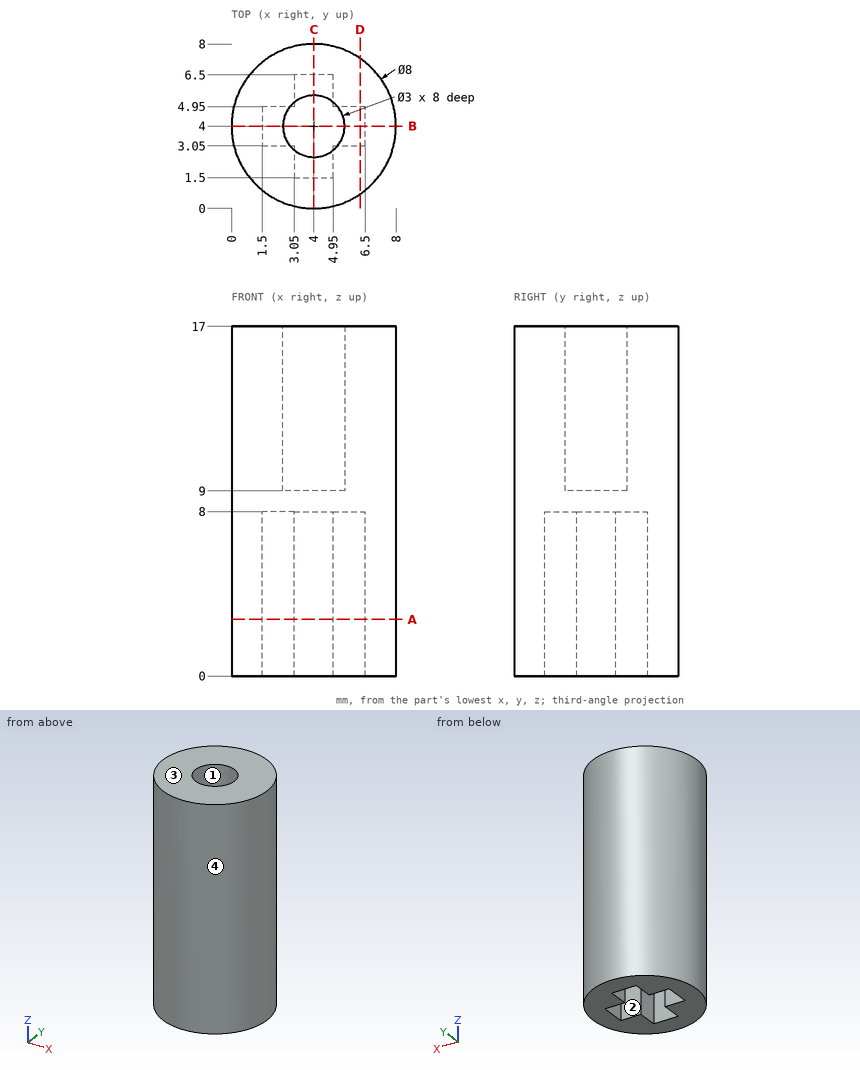
Input: dimensioned drawing with shaded views. Units: mm. Origin: part minimum x, y, z. Coordinates: 2 decimals unless noted, no trailing zeros. Write each loop counter-clockwise with the first axis right and the second up, starting at its lowest first coordinate (ties: lowest second). Pieces come first, ordered by that corner, then holes. Notation, with made-up numbers: (8, -2.75) -> (25, -2.75) arc R34 ccw to (25, 30.25) -> close; hole circle Ø6 at (54.25, 51.5). An arc over 180 degrees is marked (long way). Return JSON: item names as keys, results as strings. Group by question number.
1) Ray query, line 1 along Y through (x, z) = (4, 15.25); line 2 along X through (y, z) = (3.75, 3.5); line 3 along Y through (x, z) = (4.5, 14.25). Return the intervals inside material, ascending.
2) Contact query for flat-ended pins moving along their axis: P1, Ø1.5, axis at y = 1.5, z = 14.5, coming from the +X side; P2, Ø1.7, axis at y = 2, z = 5, coming from the -X side; P3, Ø2.5, axis at x = 4, y = 4, coming from the -Z side. Output: stop coordinate, or through.
3) Mould query, pull axis X, two halves, no side actions, for the marked faces 1, 2, 3 and 4. Classes: +X half, -X half, draft (parallel to the pull), parting line (faces both ways), or undercut.
4) Section query D-D, the plane x = 6.25. Return loops of the section in (y, z), plus the area to 3 significant figures.
5) Section query B-B, the plane y = 4. Return loops of the section in (x, z), plus the area to 3 significant figures.
6) Section query A-A, the plane z = 2.75. Return loops of the section in (x, y).
From the geometry:
{
 "1": {"line 1": "0 to 2.5, 5.5 to 8", "line 2": "0.01 to 1.5, 6.5 to 7.99", "line 3": "0.03 to 2.59, 5.41 to 7.97"},
 "2": {"P1": "x = 7.6", "P2": "x = 0.17", "P3": "z = 8"},
 "3": {"face 1": "undercut", "face 2": "undercut", "face 3": "draft", "face 4": "parting line"},
 "4": {"outline": "(0.69, 0) -> (3.05, 0) -> (3.05, 8) -> (4.95, 8) -> (4.95, 0) -> (7.31, 0) -> (7.31, 17) -> (0.69, 17) -> close", "area": "97.2 mm²"},
 "5": {"outline": "(0, 0) -> (1.5, 0) -> (1.5, 8) -> (6.5, 8) -> (6.5, 0) -> (8, 0) -> (8, 17) -> (5.5, 17) -> (5.5, 9) -> (2.5, 9) -> (2.5, 17) -> (0, 17) -> close", "area": "72.0 mm²"},
 "6": {"outline": "circle Ø8 at (4, 4); hole (1.5, 3.05) -> (3.05, 3.05) -> (3.05, 1.5) -> (4.95, 1.5) -> (4.95, 3.05) -> (6.5, 3.05) -> (6.5, 4.95) -> (4.95, 4.95) -> (4.95, 6.5) -> (3.05, 6.5) -> (3.05, 4.95) -> (1.5, 4.95) -> close"}
}
